Source: three-view drawing plus pictorial views. Frame: mm from the lowest corner of the part. Give positions to 0.01 mm unless a question says otherwise; leave off trailing zeros. Loops run counter-clockwise (first coordinate to the right, second up) from the corner with the lowest first, then second, coordinate; pieces in that order, holes last. Notation, with made-up numbers: (20.5, -26) -> (43.5, -26) arc R20 cw to (43.5, 10) -> close; hole circle Ø8 at (56, 6.25). An arc over 180 degrees is marked (long way). Answer as a JSON object with one key per item and string values. Group by question number.
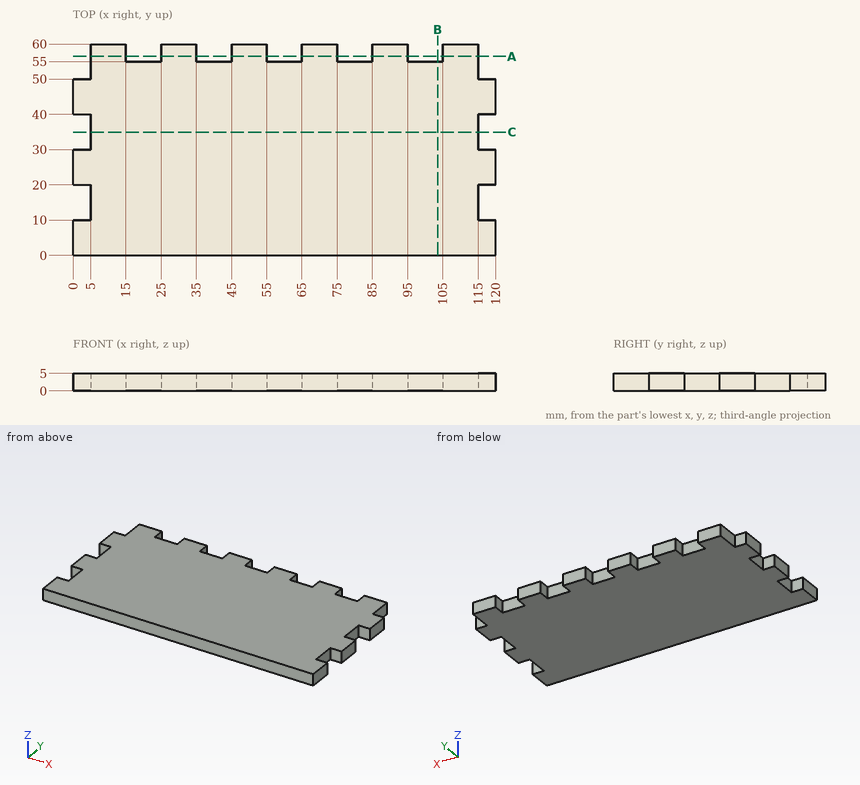
Q1. Section B-B on x = 103.5. Return the cut outline in (y, z), then the cut area to 3 significant figures.
Q2. Section A-A on y = 56.5. Return the cut outline in (x, z).
Q3. Pin query (flat end, axial travel): pin 1 Ø1.5 at (x, z) = (117.5, 2.5) entering from +Y; pin 2 Ø1.5 at (y, z) = (55.5, 3.5) entering from +X. Return the tip coordinate at first contact, or that it passes through.
Q4. Section C-C on y = 35. Return the cut outline in (x, z), then the cut area to 3 significant figures.
Q5. Ray query, probe 1 along Y at (x, z) = (79, 3); probe 2 along X at (y, z) = (12, 0.95). Return the intervals inside material, ascending.
Numbers:
{
 "1": {"outline": "(0, 0) -> (55, 0) -> (55, 5) -> (0, 5) -> close", "area": "275 mm²"},
 "2": {"outline": "(5, 0) -> (15, 0) -> (15, 5) -> (5, 5) -> close; (25, 0) -> (35, 0) -> (35, 5) -> (25, 5) -> close; (45, 0) -> (55, 0) -> (55, 5) -> (45, 5) -> close; (65, 0) -> (75, 0) -> (75, 5) -> (65, 5) -> close; (85, 0) -> (95, 0) -> (95, 5) -> (85, 5) -> close; (105, 0) -> (115, 0) -> (115, 5) -> (105, 5) -> close"},
 "3": {"pin 1": "stops at y = 50", "pin 2": "stops at x = 115"},
 "4": {"outline": "(5, 0) -> (115, 0) -> (115, 5) -> (5, 5) -> close", "area": "550 mm²"},
 "5": {"probe 1": "y = 0 to 55", "probe 2": "x = 5 to 115"}
}
